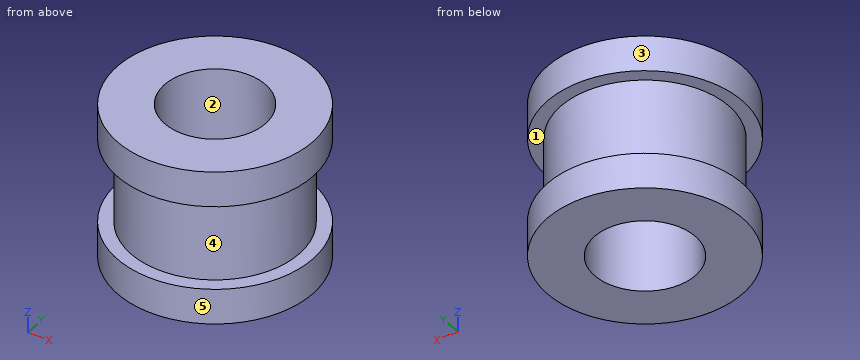
```python
from build123d import *

# Parameters (mm, degrees)
SKETCH1_R           = 2.9
BOSS_EXTRUDE1_DEPTH = 1.05
SKETCH2_R           = 2.5
BOSS_EXTRUDE2_DEPTH = 2.5
SKETCH3_R           = 1.5
CUT_EXTRUDE1_DEPTH  = 4.6


with BuildPart() as part:
    # Sketch1 → Boss-Extrude1 (new body)
    with BuildSketch(Plane.XY):
        Circle(SKETCH1_R)
    boss_extrude1 = extrude(amount=BOSS_EXTRUDE1_DEPTH)

    # Sketch2 → Boss-Extrude2 (add)
    with BuildSketch(Plane.XY.offset(1.05)):
        Circle(SKETCH2_R)
    extrude(amount=BOSS_EXTRUDE2_DEPTH)

    # Mirror1: Boss-Extrude1 across plane
    add(boss_extrude1.mirror(Plane.XY.offset(2.3)))

    # Sketch3 → Cut-Extrude1 (cut)
    with BuildSketch(Plane(origin=(0, 0, 0), x_dir=(-1, 0, 0), z_dir=(0, 0, -1))):
        Circle(SKETCH3_R)
    extrude(amount=-CUT_EXTRUDE1_DEPTH, mode=Mode.SUBTRACT)


solid = part.part
```
The model under review builds one solid part; all positions refer to its coordinate system, in mm. Face numbers are marked on the shaded views. A direction names the side the tool comes from. Round coordinates to 2 decimals unless told otherwise and drop trailing zeros. Write each loop counter-clockwise with the first axis right and the second up, starting at its lowest first coordinate (ties: lowest second). Pieces come first, ordered by that corner, then holes. Notation, with made-up numbers: M 6,6 L 55,6 A19 cw 55,36 Z; hole C -40,65 d4. An arc over 180 degrees is marked long. Use CSV: the item, a comma, the result in double quotes. Start each with the question number.
(1) For line 1 along Z through (x, y) = (-1.45, -2.25); line 2 along Y through (x, z) = (0, 1.9); line 3 along Y through (x, z) = (0, 0.9), list the stretches that pass through material, from the lowest coordinate up.
(2) We need section C-C, the plane z = 1.85. State the section outline as (x, y) points.
(3) We need section A-A, the plane y = 0. State the section outline as (x, z) points.
(4) We need section D-D, the plane y = 1.9. State the section outline as (x, z) points.
(5) Tool access review of the marked faces 4 and 5: name each direction out of +Z, -Z, +X, -X, +Y, -Y from which nothing blocks a thin tool from reaching the whole face with its end or side.
(6) Clearance check with flat-ended pins moving along their axes: P1, Ø1.5, axis at y = -0.5, z = 2.5, coming from the -X side; P2, Ø1.5, axis at x = -1, z = 1.5, coming from the -Y side. State where each tip first meets the part, or that it passes through.
(7) The part is to be moulded in two halves that separate along Y. For the marked faces 1, 2 and 3, say which applies: +Y half, -Y half, draft (parallel to the pull), parting line (faces both ways), or undercut.
Findings:
1,line 1,"0 to 1.05, 3.55 to 4.6"
1,line 2,"-2.5 to -1.5, 1.5 to 2.5"
1,line 3,"-2.9 to -1.5, 1.5 to 2.9"
2,outline,"C 0,0 d5; hole C 0,0 d3"
3,outline,"M -2.9,0 L -1.5,0 L -1.5,4.6 L -2.9,4.6 L -2.9,3.55 L -2.5,3.55 L -2.5,1.05 L -2.9,1.05 Z; M 1.5,0 L 2.9,0 L 2.9,1.05 L 2.5,1.05 L 2.5,3.55 L 2.9,3.55 L 2.9,4.6 L 1.5,4.6 Z"
4,outline,"M -2.19,0 L 2.19,0 L 2.19,1.05 L 1.62,1.05 L 1.62,3.55 L 2.19,3.55 L 2.19,4.6 L -2.19,4.6 L -2.19,3.55 L -1.62,3.55 L -1.62,1.05 L -2.19,1.05 Z"
5,face 4,"none"
5,face 5,"+Z, -Z"
6,P1,"x = -2.5"
6,P2,"y = -2.87"
7,face 1,"draft"
7,face 2,"undercut"
7,face 3,"parting line"
